Design review of the part built by this model. Coordinates are the model's own, in mm. Face numbers are marked on the shaded views. A direction names the side the tool comes from. Round coordinates to 2 decimals unless told otherwise and drop trailing zeros. Order: outer loops, then holes, each group sorted by start corner. A loop starts at its lowest first (then second) coordinate and runs counter-clockwise, first axis right, second up. Notation, with made-up numbers: (38, 47) - (87, 47) arc R8 cw to (87, 56) - close; hole circle Ø9 at (-34.75, 7). An arc over 180 degrees is marked (long way). Use CSV: the item, a comma, the result in double quotes.
from build123d import *

# Parameters (mm, degrees)
SKETCH5_W          = 15
SKETCH5_H          = 4
SKETCH6_R          = 5.5
CUT_EXTRUDE1_DEPTH = 5
SKETCH7_R          = 2.5
CUT_EXTRUDE2_DEPTH = 5
FILLET1_R          = 2
SKETCH9_R          = 3.7
CUT_EXTRUDE3_DEPTH = 2.5


with BuildPart() as part:
    # Sweep1: sweep along a path in Sketch2
    with BuildLine(Plane.XY) as sweep1_path:
        Line((-25, 0), (-2.5, 0))
        ThreePointArc((-2.5, 0), (-0.732233047, 0.732233047), (0, 2.5))
        Line((0, 2.5), (0, 25))
    # Sketch5 → Sweep1 (sweep)
    with BuildSketch(Plane(origin=(-25, 0, 0), x_dir=(0, 0, -1), z_dir=(1, 0, 0))):
        Rectangle(SKETCH5_W, SKETCH5_H)
    sweep(path=sweep1_path.line)

    # Sketch6 → Cut-Extrude1 (cut, through all)
    with BuildSketch(Plane(origin=(0, 2, 0), x_dir=(1, 0, 0), z_dir=(0, 1, 0))):
        with Locations((-17.5, 0)):
            Circle(SKETCH6_R)
    extrude(amount=-CUT_EXTRUDE1_DEPTH, mode=Mode.SUBTRACT)

    # Sketch7 → Cut-Extrude2 (cut, through all)
    with BuildSketch(Plane.ZY.offset(2)):
        with Locations((0, 17.5)):
            Circle(SKETCH7_R)
    extrude(amount=-CUT_EXTRUDE2_DEPTH, mode=Mode.SUBTRACT)

    # Fillet1
    fillet1_edges = [part.edges().sort_by_distance(p)[0] for p in [
        (-25, 0, 7.5),
        (0, 25, -7.5),
        (0, 25, 7.5),
        (-25, 0, -7.5),
    ]]
    fillet(fillet1_edges, radius=FILLET1_R)

    # Sketch9 → Cut-Extrude3 (cut)
    with BuildSketch(Plane.ZY.offset(2)):
        with Locations((0, 17.5)):
            Circle(SKETCH9_R)
    extrude(amount=-CUT_EXTRUDE3_DEPTH, mode=Mode.SUBTRACT)


solid = part.part
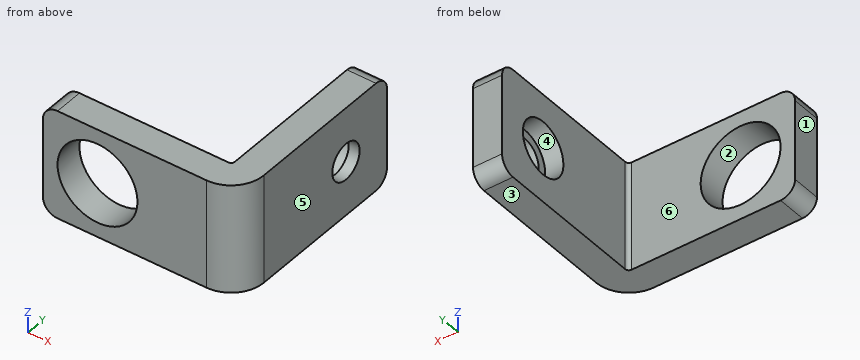
1) For the marked faces 5 and 6, list the 3-axis set-ups (+Z, -Z, +X, -X, +Y, -Y) from which the entire face can be reached by the end or side of a thin tool; tool diameter is ignored.
Data:
face 5,"+Z, -Z, +X, +Y, -Y"
face 6,"+Z, -Z, -X, +Y"
2) We need section C-C (y = 17.5). Give the boundary of the cut face in (x, z), then the cut area to 3 significant figures.
Data:
outline,"(-2, -7.5) - (2, -7.5) - (2, -2.5) - (0.5, -2.5) - (0.5, -3.7) - (-2, -3.7) - close; (-2, 3.7) - (0.5, 3.7) - (0.5, 2.5) - (2, 2.5) - (2, 7.5) - (-2, 7.5) - close"
area,"34.0 mm2"
3) We need section B-B (z = 0). Give the boundary of the cut face in (x, y), then the cut area to 3 significant figures.
Data:
outline,"(-25, -2) - (-23, -2) - (-23, 2) - (-25, 2) - close; (-12, -2) - (-2.5, -2) arc R4.5 ccw to (2, 2.5) - (2, 15) - (0.5, 15) - (0.5, 13.8) - (-2, 13.8) - (-2, 2.5) arc R0.5 cw to (-2.5, 2) - (-12, 2) - close; (-2, 21.2) - (0.5, 21.2) - (0.5, 20) - (2, 20) - (2, 25) - (-2, 25) - close"
area,"126 mm2"
4) The part is to be moulded in two halves that separate along Z. For the marked faces 1, 2, 3 and 4, say which applies: +Z half, -Z half, draft (parallel to the pull), parting line (faces both ways), or undercut.
Data:
face 1,"draft"
face 2,"undercut"
face 3,"-Z half"
face 4,"undercut"
5) Insertion check: pin 1 Ø7.5 at (y, z) = (11.5, -0.5) entering from -X. The pin has a flat end and moves straight along its axis. Give the tip position at first contact, or say it passes through.
Data:
pin 1,"stops at x = -2"
6) We need section A-A (x = -17.5). Give the boundary of the cut face in (y, z), then the cut area to 3 significant figures.
Data:
outline,"(-2, -7.5) - (2, -7.5) - (2, -5.5) - (-2, -5.5) - close; (-2, 5.5) - (2, 5.5) - (2, 7.5) - (-2, 7.5) - close"
area,"16.0 mm2"
7) We need section D-D (z = 4.5). Give the boundary of the cut face in (x, y), then the cut area to 3 significant figures.
Data:
outline,"(-25, -2) - (-20.66, -2) - (-20.66, 2) - (-25, 2) - close; (-14.34, -2) - (-2.5, -2) arc R4.5 ccw to (2, 2.5) - (2, 25) - (-2, 25) - (-2, 2.5) arc R0.5 cw to (-2.5, 2) - (-14.34, 2) - close"
area,"170 mm2"
8) To check wall thickness, follow L1, parallel to Z at x = -17.5, y = 1.05; L2, parallel to Y at x = -12.5, z = -4. State the ranges of each line that lie inside material, in increasing order. Write a range as from..to.
Data:
L1,"z = -7.5..-5.5, 5.5..7.5"
L2,"y = -2..2"
